from build123d import *

# Parameters (mm, degrees)
BOSS_EXTRU_1_DEPTH      = 10
ESQUISSE2_W             = 100
ESQUISSE2_H             = 10
ESQUISSE2_W_2           = 10
ESQUISSE2_H_2           = 50
ESQUISSE2_W_3           = 50
ENL_V_MAT_EXTRU_1_DEPTH = 10


with BuildPart() as part:
    # Esquisse1 → Boss.-Extru.1 (new body)
    with BuildSketch(Plane.XY):
        Polygon((-310, 0), (0, 490.204039151), (310, 0), (75, 0), (75, -120), (-75, -120), (-75, 0), align=None)
    extrude(amount=BOSS_EXTRU_1_DEPTH)

    # Esquisse2 → Enlèv. mat.-Extru.1 (cut)
    with BuildSketch(Plane.XY.offset(10)):
        Polygon((-269.913793103, 63.388453338), (-261.461999325, 58.043625752), (-208.013723463, 142.561563537), (-216.465517241, 147.906391123), align=None)
        Polygon((-181.724137931, 202.843050683), (-173.272344153, 197.498223097), (-119.82406829, 282.016160882), (-128.275862069, 287.360988468), align=None)
        Polygon((-93.534482759, 342.297648028), (-85.08268898, 336.952820442), (-31.634413118, 421.470758226), (-40.086206897, 426.815585813), align=None)
        Polygon((208.013723463, 142.561563537), (216.465517241, 147.906391123), (269.913793103, 63.388453338), (261.461999325, 58.043625752), align=None)
        Polygon((31.634413118, 421.470758226), (40.086206897, 426.815585813), (93.534482759, 342.297648028), (85.08268898, 336.952820442), align=None)
        Polygon((119.82406829, 282.016160882), (128.275862069, 287.360988468), (181.724137931, 202.843050683), (173.272344153, 197.498223097), align=None)
        with Locations((-160, 5)):
            Rectangle(ESQUISSE2_W, ESQUISSE2_H)
        with Locations((160, 5)):
            Rectangle(ESQUISSE2_W, ESQUISSE2_H)
        with Locations((-70, -60)):
            Rectangle(ESQUISSE2_W_2, ESQUISSE2_H_2)
        with Locations((70, -60)):
            Rectangle(ESQUISSE2_W_2, ESQUISSE2_H_2)
        with Locations((0, -115)):
            Rectangle(ESQUISSE2_W_3, ESQUISSE2_H)
    extrude(amount=-ENL_V_MAT_EXTRU_1_DEPTH, mode=Mode.SUBTRACT)


solid = part.part
Model file for the job. Use its own axes, mm. Coordinates: 2 decimals unless noted, no trailing zeros. Order: outer loops, then holes, each group sorted by start corner. A loop starts at its lowest first (then second) coordinate and runs counter-clockwise, first axis right, second up. Notation, with made-up numbers: (55.25, 5.5) -> (109.25, 5.5) arc R15 ccw to (109.25, 31.5) -> close; hole circle Ø7 at (49.5, -26). An arc over 180 degrees is marked (long way). Return JSON: item names as keys, results as strings. Group by question number.
Item 1: Saw through at A-A on y = -62. Write the cut outline in (x, z), then the cut area to 3 significant figures.
Item 2: Saw through at B-B on x = -58. Write the cut outline in (y, z).
Item 3: Flat gauge pins, fed straight in: P1, Ø3, axis at y = 6, z = 4.5, coming from the -X side; P2, Ø5, axis at x = -11, z = 3, coming from the -Y side; P3, Ø5, axis at x = 148, z = 1, coming from the +Y side. Where does each tip first touch, or does it go through?
Item 4: Wall check: line 1 along X through (y, z) = (198, 4); line 2 along X through (y, z) = (-29, 6.25); line 3 along Y through (x, z) = (69.5, 3.5). Give the ranges that are in metal, low to high. Write a range as [from, to].
Values found:
{
 "1": {"outline": "(-65, 0) -> (65, 0) -> (65, 10) -> (-65, 10) -> close", "area": "1,300 mm2"},
 "2": {"outline": "(-120, 0) -> (379.78, 0) -> (379.78, 10) -> (-120, 10) -> close"},
 "3": {"P1": "stops at x = -307.15", "P2": "stops at y = -110", "P3": "stops at y = 241.41"},
 "4": {"line 1": "x = [-184.79, -174.07], [-172.96, 172.96], [174.07, 184.79]", "line 2": "x = [-75, 75]", "line 3": "y = [-120, -85], [-35, 361.59]"}
}
